Input: part model. Units: mm. Frame: model coordinates. A direction names the side the tool comes from. Coordinates: 2 decimals unless noted, no trailing zeros. Write each loop counter-clockwise with the first axis right and the second up, starting at its lowest first coordinate (ties: lowest second). Pieces come first, ordered by that corner, then holes. Notation, with made-up numbers: (55.5, 0) - (107.5, 0) arc R19 ccw to (107.5, 23) - close; hole circle Ø5 at (-2.5, 83.5). An arc over 180 degrees is marked (long way). Use a Markdown table: item, result. Add a question column.
Q1. Section query A-A (x = 9.6). Return the cut outline in (y, z).
Q2. Pin query (flat end, axial travel): P1, Ø10, axis at y = 33, z = 5, coming from the -X side; P2, Ø5.5, axis at x = 15, y = 5, coming from the +Z side; P3, Ø2, axis at x = 21.5, z = 0.5, coming from the +Y side. Return the tip coordinate at first contact, or that it passes through.
Q3. Section query D-D (y = 1.65). Return the cut outline in (x, z) (1 decimal), then the cut area to 3 significant figures.
Q4. Section query B-B (z = -4). Return the cut outline in (x, y).
Q5. Section query C-C (y = 9). Return the cut outline in (x, z) (1 decimal).
Q6. Set-up query: faces 4 (the face through (17, 3, 2)), 5 (the face through (17, -1, -8)), 6 (the face through (-38, 47, 23.825)). Return all of +Z, -Z, +X, -X, +Y, -Y with unobstructed straight access to the full face (end or side cutting, diameter ignored); none if empty.
Q7. Mould query, pull axis X, two halves, no side actions, for faces 1 (the face through (-37, 0, 7)), 2 (the face through (17.784, 16.161, 0.986)), 3 (the face through (35, 6, -2)). Classes: released by +X, released by -X, zero draft, split by the parting line, or undercut.
Q8. Material intervals for probe 1 along Y at (x, z) = (16.9, 0.55); probe 2 along Y at (x, z) = (26, 1); probe 3 along Z at (x, y) = (-54, 13) (3 decimals), sorted ascending. Write a range as from..to.
from build123d import *

# Parameters (mm, degrees)
SKETCH1_W            = 35
SKETCH1_H            = 17
BOSS_EXTRUDE1_DEPTH  = 2
M2_CLEARANCE_HOLE1_D = 2.4
SKETCH6_W            = 35
SKETCH6_H            = 10
BOSS_EXTRUDE2_DEPTH  = 2
SKETCH7_W            = 33
SKETCH7_H            = 10
CUT_EXTRUDE1_DEPTH   = 41.174618853
M2_CLEARANCE_HOLE2_D = 2.4
SKETCH10_W           = 36.5
SKETCH10_H           = 2
BOSS_EXTRUDE3_DEPTH  = 72.237500028
BOSS_EXTRUDE4_DEPTH  = 50
CUT_EXTRUDE2_DEPTH   = 69.237500028
BOSS_EXTRUDE5_DEPTH  = 1
FILLET1_R            = 2.54
SKETCH15_R           = 2.38125
CUT_EXTRUDE3_DEPTH   = 93.539786229


with BuildPart() as part:
    # Sketch1 → Boss-Extrude1 (new body)
    with BuildSketch(Plane.XY):
        with Locations((17.5, 8.5)):
            Rectangle(SKETCH1_W, SKETCH1_H)
    extrude(amount=BOSS_EXTRUDE1_DEPTH)

    # M2 Clearance Hole1 (through all)
    with Locations(Plane.XY.offset(2)):
        with Locations((16.9, 15.35), (30, 15.35), (30, 1.65), (16.9, 1.65)):
            Hole(M2_CLEARANCE_HOLE1_D / 2)

    # Sketch6 → Boss-Extrude2 (add)
    with BuildSketch(Plane.XZ):
        with Locations((17.5, -3)):
            Rectangle(SKETCH6_W, SKETCH6_H)
    extrude(amount=BOSS_EXTRUDE2_DEPTH)

    # Sketch7 → Cut-Extrude1 (cut, through all)
    with BuildSketch(Plane.XY.offset(2)):
        with Locations((17.5, 8.5)):
            Rectangle(SKETCH7_W, SKETCH7_H)
    extrude(amount=-CUT_EXTRUDE1_DEPTH, mode=Mode.SUBTRACT)

    # M2 Clearance Hole2 (through all)
    with Locations(Plane(origin=(0, 0, 0), x_dir=(1, 0, 0), z_dir=(0, 1, 0))):
        with Locations((30, 4), (5, 4)):
            Hole(M2_CLEARANCE_HOLE2_D / 2)

    # Sketch10 → Boss-Extrude3 (add)
    with BuildSketch(Plane.ZY):
        with Locations((7.075, -1)):
            Rectangle(SKETCH10_W, SKETCH10_H)
    extrude(amount=BOSS_EXTRUDE3_DEPTH)

    # Sketch11 → Boss-Extrude4 (add)
    with BuildSketch(Plane(origin=(0, 0, 0), x_dir=(1, 0, 0), z_dir=(0, 1, 0))):
        Polygon((0, -25.325), (-72.237500028, -25.325), (-72.237500028, -22.325), (-69.237500028, -22.325), (-3, -22.325), (-3, 8.175), (-69.237500028, 8.175), (-72.237500028, 8.175), (-72.237500028, 11.175), (0, 11.175), align=None)
    extrude(amount=BOSS_EXTRUDE4_DEPTH)

    # Sketch12 → Cut-Extrude2 (cut)
    with BuildSketch(Plane.ZY.offset(72.237500028)):
        Polygon((23.825, 48.5), (22.325, 48.5), (-8.175, 48.5), (-9.675, 48.5), (-9.675, 45.5), (-8.175, 45.5), (22.325, 45.5), (23.825, 45.5), align=None)
    extrude(amount=-CUT_EXTRUDE2_DEPTH, mode=Mode.SUBTRACT)

    # Sketch14 → Boss-Extrude5 (add)
    with BuildSketch(Plane(origin=(35, 0, 0), x_dir=(0, 0, -1), z_dir=(1, 0, 0))):
        Polygon((8, 0), (0, 17), (0, 0), align=None)
    extrude(amount=-BOSS_EXTRUDE5_DEPTH)

    # Fillet1
    # the kernel refuses this fillet: 2.54 mm, written as the material it takes off along each edge
    with BuildSketch(Plane(origin=(0, 56.35, 25.325), x_dir=(0, 0, -1), z_dir=(0, -1, 0)), Plane(origin=(-72.237500028, 56.35, 25.325), x_dir=(1, 0, 0), z_dir=(0, -1, 0)), Plane(origin=(-72.237500028, -8.35, -11.175), x_dir=(1, 0, 0), z_dir=(0, 1, 0)), Plane(origin=(0, -8.35, -11.175), x_dir=(0, 0, 1), z_dir=(0, 1, 0))) as fillet1_piece_1:
        with BuildLine():
            CenterArc((FILLET1_R, -FILLET1_R), FILLET1_R, 90, 90)
            Line((0, -FILLET1_R), (0, 0))
            Line((0, 0), (FILLET1_R, 0))
        make_face()
    extrude(amount=64.7, mode=Mode.SUBTRACT)

    # Sketch15 → Cut-Extrude3 (cut, through all)
    with BuildSketch(Plane.XZ.offset(2)):
        with Locations(Location((9.6, -4, 0), (0, 0, 270))):
            Circle(SKETCH15_R)
    extrude(amount=-CUT_EXTRUDE3_DEPTH, mode=Mode.SUBTRACT)


solid = part.part
Values follow:
| question | item | result |
|---|---|---|
| 1 | outline | (-2, -8) - (0, -8) - (0, -6.38) - (-2, -6.38) - close; (-2, -1.62) - (0, -1.62) - (0, 0) - (3.5, 0) - (3.5, 2) - (-2, 2) - close; (13.5, 0) - (17, 0) - (17, 2) - (13.5, 2) - close |
| 2 | P1 | x = -3 |
| 2 | P2 | z = 2 |
| 2 | P3 | y = 17 |
| 3 | outline | (-72.2, -8.6) arc R2.5 ccw to (-69.7, -11.2) - (-2.5, -11.2) arc R2.5 ccw to (0, -8.6) - (0, 0) - (15.7, 0) - (15.7, 2) - (0, 2) - (0, 22.8) arc R2.5 ccw to (-2.5, 25.3) - (-69.7, 25.3) arc R2.5 ccw to (-72.2, 22.8) - (-72.2, 22.3) - (-3, 22.3) - (-3, -8.2) - (-72.2, -8.2) - close; (18.1, 0) - (28.8, 0) - (28.8, 2) - (18.1, 2) - close; (31.2, 0) - (34, 0) - (34, -7.2) - (35, -7.2) - (35, 2) - (31.2, 2) - close |
| 3 | area | 587 mm2 |
| 4 | outline | (-72.24, -2) - (3.8, -2) - (3.8, 0) - (0, 0) - (0, 50) - (-3, 50) - (-3, 0) - (-72.24, 0) - close; (6.2, -2) - (7.22, -2) - (7.22, 0) - (6.2, 0) - close; (11.98, -2) - (28.8, -2) - (28.8, 0) - (11.98, 0) - close; (31.2, -2) - (35, -2) - (35, 8.5) - (34, 8.5) - (34, 0) - (31.2, 0) - close |
| 5 | outline | (-72.2, -8.6) arc R2.5 ccw to (-69.7, -11.2) - (-2.5, -11.2) arc R2.5 ccw to (0, -8.6) - (0, 0) - (1, 0) - (1, 2) - (0, 2) - (0, 22.8) arc R2.5 ccw to (-2.5, 25.3) - (-69.7, 25.3) arc R2.5 ccw to (-72.2, 22.8) - (-72.2, 22.3) - (-3, 22.3) - (-3, -8.2) - (-72.2, -8.2) - close; (34, -3.8) - (35, -3.8) - (35, 2) - (34, 2) - close |
| 6 | face 4 | +Z, +X, +Y, -Y |
| 6 | face 5 | -Z, +X, +Y, -Y |
| 6 | face 6 | -X |
| 7 | face 1 | zero draft |
| 7 | face 2 | undercut |
| 7 | face 3 | released by +X |
| 8 | probe 1 | -2..0.45, 2.85..3.5, 13.5..14.15, 16.55..17 |
| 8 | probe 2 | -2..3.5, 13.5..17 |
| 8 | probe 3 | -11.175..-8.175, 22.325..25.325 |
